```python
from build123d import *

# Parameters (mm, degrees)
F0_R     = 200
F1_DEPTH = 39
F2_R     = 6
F3_DEPTH = 25


with BuildPart() as f1:
    # F0 (on Top) → F1 (new body)
    with BuildSketch(Plane.XY):
        Circle(F0_R)
    extrude(amount=F1_DEPTH)

    # F2 (on face) → F3 (cut)
    with BuildSketch(Plane(origin=(0, 0, 0), x_dir=(1, 0, 0), z_dir=(0, 0, -1))):
        with Locations((110.25921, 108.939922)):
            Circle(F2_R)
        with Locations((110.25921, -108.939922)):
            Circle(F2_R)
        with Locations((-110.25921, -108.939922)):
            Circle(F2_R)
        with Locations((-110.25921, 108.939922)):
            Circle(F2_R)
    extrude(amount=-F3_DEPTH, mode=Mode.SUBTRACT)


solid = f1.part
```
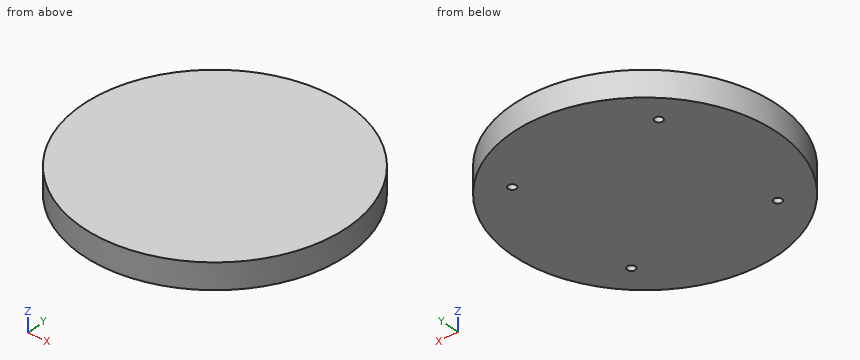
Part model, mm, in its own coordinate system. Give positions to 0.01 mm unless a question says otherwise; leave off trailing zeros. Order: outer loops, then holes, each group sorted by start corner. A loop starts at its lowest first (then second) coordinate and runs counter-clockwise, first axis right, second up. Notation, with made-up numbers: M -31.75,-25.5 L 11.25,-25.5 A30 cw 11.25,-3.5 Z; hole C 24,87 d4. An arc over 180 degrees is marked long. Use a Markdown table: item, result. Add a question column.
(1) Drop flat-ended pins along their axis: P1, Ø6, axis at x = 110, y = -110, coming from the -Z side; P2, Ø5, axis at x = 27.5, z = 29.5, coming from the +Y side; P3, Ø8, axis at x = 102, z = 27, coming from the -Y side. Give the stop position or say it passes through.
(2) Probe line 1 along Y through (x, z) = (181, 15); line 2 along Y through (x, z) = (-17, 33); line 3 along X through (y, z) = (115.5, 6.5). List the from-to ranges inside material, lowest first. Write a range as [from, to].
(3) Saw through at B-B, the plane y = 163.5. Give the cut face in (x, z).
(4) Saw through at A-A, the plane z = 15. Give the cut face in (x, y), and give its area (3 significant figures).
Answer key:
| question | item | result |
|---|---|---|
| 1 | P1 | z = 25 |
| 1 | P2 | y = 198.43 |
| 1 | P3 | y = -174.34 |
| 2 | line 1 | [-85.08, 85.08] |
| 2 | line 2 | [-199.28, 199.28] |
| 2 | line 3 | [-163.28, 163.28] |
| 3 | outline | M -115.19,0 L 115.19,0 L 115.19,39 L -115.19,39 Z |
| 4 | outline | C 0,0 d400; hole C -110.26,-108.94 d12; hole C -110.26,108.94 d12; hole C 110.26,-108.94 d12; hole C 110.26,108.94 d12 |
| 4 | area | 125,000 mm^2 |
